Autodesk Inventor part; units mm, degrees
ref_plane "Work Plane1" through (0, 0, 0) normal (0, 1, 0) x (-1, 0, 0)
ref_plane "Work Plane2" through (0, 0, 0) normal (0, 1, 0) x (-1, 0, 0)
ref_plane "Work Plane3" through (0, 0, 0) normal (1, 0, 0) x (0, 1, 0)
sketch "Sketch1" plane through (0, 0, 0) normal (0, 0, 1) x (1, 0, 0)
  circle A0 centre (0, 0) radius 18.0975
  dimension "d0" = 36.195
extrude "Extrusion1" add sketch "Sketch1" along normal blind 19.685
chamfer "Chamfer1" distance 0.7937 angle 45 1 edges at (-18.0975, 0, 19.685)
sketch "Sketch2" plane through (0, 0, 0) normal (0, 0, -1) x (-1, 0, 0)
  circle A0 centre (0, 0) radius 18.0975
  circle A1 centre (0, 0) radius 16.8275
  dimension "d6" = 33.655
extrude "Extrusion2" add sketch "Sketch2" along normal blind 1.905 contours A1
ref_plane "Work Plane1" through (0, 0, 0) normal (0, 1, 0) x (-1, 0, 0)
sketch "Sketch3" plane through (0, 0, 0) normal (0, 1, 0) x (-1, 0, 0)
  line L0 (-18.0975, 0) -> (18.0975, 0)
  line L1 (18.0975, 18.8913) -> (-18.0975, 18.8913)
  line L2 (18.0975, 0) -> (18.0975, 18.8913)
  line L3 (-18.0975, 0) -> (-18.0975, 18.8913)
  circle A0 centre (0, 9.4456) radius 5.3975
  point P0 (0, 0)
  dimension "d10" = 10.795
extrude "Extrusion3" cut sketch "Sketch3" against normal mid plane 76.2 contours A0
ref_plane "Work Plane2" through (0, 0, 0) normal (0, 1, 0) x (-1, 0, 0)
sketch "Sketch4" plane through (0, 0, 0) normal (0, 1, 0) x (-1, 0, 0)
  point P0 (0, 0)
ref_plane "Work Plane3" through (0, 0, 0) normal (1, 0, 0) x (0, 1, 0)
sketch "Sketch5" plane through (0, 0, 0) normal (1, 0, 0) x (0, 1, 0)
  line L0 (18.0975, 0) -> (18.0975, 18.8913)
  line L1 (-18.0975, 0) -> (-18.0975, 18.8913)
  line L2 (-18.0975, 0) -> (18.0975, 0)
  line L3 (-17.3038, 19.685) -> (17.3038, 19.685)
  circle A0 centre (0, 9.4456) radius 5.3975
  point P0 (0, 0)
  dimension "d15" = 10.795
extrude "Extrusion4" cut sketch "Sketch5" against normal mid plane 76.2
thread "Thread1"
thread "Thread2"
thread "Thread3"
thread "Thread4"
properties part number "Regulator Base 1764"
The listing builds one solid part. Answer for the finished solid, in the listing's coordinates (mm). A direction names the side the tool comes from. Round coordinates to 2 decimals unless told otherwise and drop trailing zeros. Write each loop counter-clockwise with the first axis right and the second up, starting at its lowest first coordinate (ties: lowest second). Pieces come first, ordered by that corner, then holes. Notation, with made-up numbers: (-13.75, 48) -> (43.25, 48) arc R22 cw to (43.25, 67) -> close; hole circle Ø5 at (-10.5, 43.25). An arc over 180 degrees is marked (long way). Answer as a JSON object with one key per item and string values. Group by question number.
Q1. Which of the six approach directions +Z, -Z, +X, -X, +Y, -Y give full straight-line access (tool end or side, diameter ignored) to faces 1 (the face through (11, -13, 0)), 2 (the face through (5.392, -10.934, 9.683))?
Q2. Section A-A (z = 5.5) is taken. Write down the section's boundary in (x, y) (1 decimal).
Q3. Straight lines are drawn through the part: line 1 along Z through (x, y) = (0, -12.25) (3 decimals); line 2 along X through (y, z) = (-11.5, 11); line 3 along Y through (x, z) = (-8, 14.25). For each, find the intervals that lie inside material, in ascending order.
Q4. Section B-B (z = 13) is taken. Write down the section's boundary in (x, y) (1 decimal).
Q5. Determine the mould class of faces 3 (the face through (3.648, 16.427, -0.939)), 4 (the face through (0, 0, 19.685)), 5 (the face through (11.186, 5.148, 11.067)) for opening direction Z: pulls with the +Z half, pulls with the -Z half, needs draft (parallel to the pull), parting line crosses it, or undercut.
Q6. Section C-C (z = 17) is taken. Write down the section's boundary in (x, y) (1 decimal), plus the area to 3 significant figures.
Q7. Each of these flat-tipped pins is pushed along its axis until it touches: pin 1 Ø1.5 at (y, z) = (-2, 5) entering from -X; pin 2 Ø1 at (y, z) = (-6.5, 14.5) entering from -X; pin 3 Ø10 at (y, z) = (-7.5, 14) entering from +X; pin 4 Ø8.5 at (x, z) = (0, 9.45) entering from -Y. Where does it stop, or does it pass through?
Check values:
{
 "1": {"face 1": "-Z", "face 2": "+Y, -Y"},
 "2": {"outline": "(-17.7, -3.7) arc R18.1 ccw to (-3.7, -17.7) -> (-3.7, -3.7) -> close; (-17.7, 3.7) -> (-3.7, 3.7) -> (-3.7, 17.7) arc R18.1 ccw to start; (3.7, -17.7) arc R18.1 ccw to (17.7, -3.7) -> (3.7, -3.7) -> close; (3.7, 3.7) -> (17.7, 3.7) arc R18.1 ccw to (3.7, 17.7) -> close"},
 "3": {"line 1": "-1.905 to 4.048, 14.843 to 19.685", "line 2": "-13.97 to -5.17, 5.17 to 13.97", "line 3": "-16.23 to -2.46, 2.46 to 16.23"},
 "4": {"outline": "(-17.6, -4.1) arc R18.1 ccw to (-4.1, -17.6) -> (-4.1, -4.1) -> close; (-17.6, 4.1) -> (-4.1, 4.1) -> (-4.1, 17.6) arc R18.1 ccw to start; (4.1, -17.6) arc R18.1 ccw to (17.6, -4.1) -> (4.1, -4.1) -> close; (4.1, 4.1) -> (17.6, 4.1) arc R18.1 ccw to (4.1, 17.6) -> close"},
 "5": {"face 3": "needs draft", "face 4": "pulls with the +Z half", "face 5": "undercut"},
 "6": {"outline": "circle Ø36.2 at (0, 0)", "area": "1,030 mm^2"},
 "7": {"pin 1": "x = -18.02", "pin 2": "x = -17.07", "pin 3": "x = 17.92", "pin 4": "through"}
}
